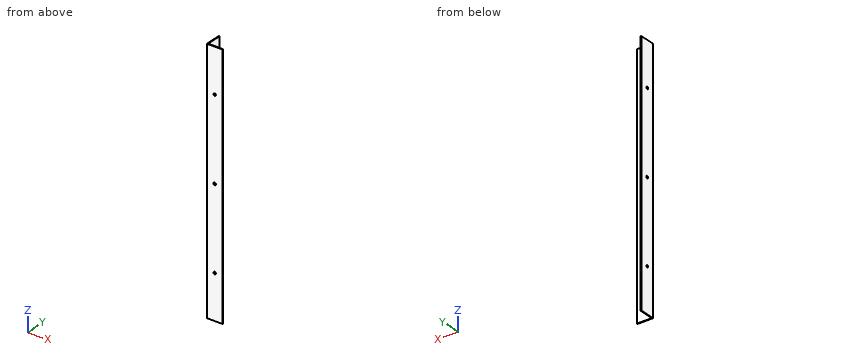
```python
from build123d import *

# Parameters (mm, degrees)
BOSS_EXTRUDE1_DEPTH          = 508
F_10_0_1935_DIAMETER_HOLE2_D = 4.9149
F_10_0_1935_DIAMETER_HOLE4_D = 4.9149


with BuildPart() as part:
    # Sketch2 → Boss-Extrude1 (new body)
    with BuildSketch(Plane.XY):
        Polygon((0, 0), (0, 31.75), (1.5875, 31.75), (1.5875, 1.5875), (31.75, 1.5875), (31.75, 0), align=None)
    extrude(amount=BOSS_EXTRUDE1_DEPTH)

    # #10 (0.1935) Diameter Hole2 (through all)
    with Locations(Plane.ZY):
        with Locations((419.1, 15.875), (88.9, 15.875), (254, 15.875)):
            Hole(F_10_0_1935_DIAMETER_HOLE2_D / 2)

    # #10 (0.1935) Diameter Hole4 (through all)
    with Locations(Plane(origin=(0, 0, 0), x_dir=(-1, 0, 0), z_dir=(0, -1, 0))):
        with Locations((-15.875, -419.1), (-15.875, -254), (-15.875, -88.9)):
            Hole(F_10_0_1935_DIAMETER_HOLE4_D / 2)


solid = part.part
```
Input: part model. Units: mm. Frame: model coordinates. Round coordinates to 2 decimals unless told otherwise and drop trailing zeros. Write each loop counter-clockwise with the first axis right and the second up, starting at its lowest first coordinate (ties: lowest second). Pieces come first, ordered by that corner, then holes. Notation, with made-up numbers: (17, 81) - (46, 81) arc R19 cw to (46, 105) - close; hole circle Ø2 at (50, 44). An arc over 180 degrees is marked (long way). Write item = value, one per line.
(1) Contact query for flat-ended pins moving along their axis: pin 1 Ø6.5 at (y, z) = (15.875, 88.9) entering from -X; pin 2 Ø1 at (y, z) = (24.5, 205.5) entering from +X; pin 3 Ø12 at (x, z) = (21, 435.5) entering from +Y. Output: stop coordinate, or through.
Geometry check:
pin_1 = 0
pin_2 = 1.59
pin_3 = 1.59
(2) Material intervals for probe 1 along Y at (x, z) = (1, 88.9); probe 2 along X at (y, z) = (16.5, 72), sorted ascending.
Geometry check:
probe_1 = 0 to 13.42, 18.33 to 31.75
probe_2 = 0 to 1.59
(3) Section query B-B on x = 26.5. Output: boundary loops of the cut face in (y, z).
Geometry check:
outline = (0, 0) - (1.59, 0) - (1.59, 508) - (0, 508) - close
(4) Section query A-A on z = 204. Output: boundary loops of the cut face in (x, y), then the cut area to 3 significant figures.
Geometry check:
outline = (0, 0) - (31.75, 0) - (31.75, 1.59) - (1.59, 1.59) - (1.59, 31.75) - (0, 31.75) - close
area = 98.3 mm^2
